from build123d import *

# Parameters (mm, degrees)
SKETCH1_W               = 20.32
SKETCH1_H               = 23.8125
BOSS_EXTRUDE1_DEPTH     = 3
SKETCH3_R               = 1.500000048
CUT_EXTRUDE1_DEPTH      = 84.279291716
CUT_EXTRUDE2_DEPTH      = 23.075453704
CUT_EXTRUDE2_DEPTH_BACK = 23.075453704
SKETCH2_R               = 78.359
SKETCH4_W               = 22.86
SKETCH4_H               = 20.306074834
CUT_EXTRUDE3_DEPTH      = 12.3825
SKETCH9_W               = 8
SKETCH9_H               = 3.175
BOSS_EXTRUDE2_DEPTH     = 10.16
BOSS_EXTRUDE3_DEPTH     = 1.27
FILLET7_R               = 5.715
FILLET8_R               = 1.27
FILLET9_R               = 1.27


# Some blends are built 0.0001 mm under size
with BuildPart() as part:
    # Sketch1 → Boss-Extrude1 (new body)
    with BuildSketch(Plane(origin=(0, 0, 0), x_dir=(1, 0, 0), z_dir=(0, 1, 0))):
        with Locations((0, -7.46125)):
            Rectangle(SKETCH1_W, SKETCH1_H)
        Polygon((3.9, -10.985), (6, -10.985), (6, -13.985), (2.999999969, -13.985), (2.999999969, -17.16), (-2.999999969, -17.16), (-2.999999969, -13.985), (-6, -13.985), (-6, -10.985), (-3.9, -10.985), (-3.9, -6.985), (3.9, -6.985), align=None, mode=Mode.SUBTRACT)
    extrude(amount=BOSS_EXTRUDE1_DEPTH)

    # Sketch3 → Cut-Extrude1 (cut, through all)
    with BuildSketch(Plane(origin=(-5.581860717, -76.451458097, 0), x_dir=(0, 0, 1), z_dir=(0.07281799962939917, 0.9973452456045363, 0))):
        with Locations(Location((0, 5.59671863, 0), (0, 0, 270))):
            Circle(SKETCH3_R)
    cut_extrude1 = extrude(amount=CUT_EXTRUDE1_DEPTH, mode=Mode.SUBTRACT)

    # Mirror1: Cut-Extrude1 across plane
    add(cut_extrude1.mirror(Plane(origin=(0, 0, 0), x_dir=(0, 0, 1), z_dir=(1, 0, 0))), mode=Mode.SUBTRACT)

    # Sketch2 → Cut-Extrude2 (cut, two sides: drawn at the far end of the back side and taken through both)
    with BuildSketch(Plane.XY.offset(-CUT_EXTRUDE2_DEPTH_BACK)):
        with Locations((0, -76.858999952)):
            Circle(SKETCH2_R)
    extrude(amount=CUT_EXTRUDE2_DEPTH + CUT_EXTRUDE2_DEPTH_BACK, mode=Mode.SUBTRACT)

    # Sketch4 → Cut-Extrude3 (cut)
    with BuildSketch(Plane.XY.offset(19.3675)):
        with Locations((-1.27, 10.991574627)):
            Rectangle(SKETCH4_W, SKETCH4_H)
    extrude(amount=-CUT_EXTRUDE3_DEPTH, mode=Mode.SUBTRACT)

    # Sketch9 → Boss-Extrude2 (add)
    with BuildSketch(Plane(origin=(0, 3, 0), x_dir=(1, 0, 0), z_dir=(0, 1, 0))):
        with Locations((0, -5.3975)):
            Rectangle(SKETCH9_W, SKETCH9_H)
    extrude(amount=BOSS_EXTRUDE2_DEPTH)

    # Sketch10 → Boss-Extrude3 (add, symmetric)
    with BuildSketch(Plane(origin=(0, 0, 0), x_dir=(0, 0, -1), z_dir=(1, 0, 0))):
        Polygon((-3.81, 13.16), (4.445, 3), (-3.81, 3), align=None)
    extrude(amount=BOSS_EXTRUDE3_DEPTH, both=True)

    # Fillet7
    fillet7_edges = [part.edges().sort_by_distance(p)[0] for p in [
        (-10.16, 1.919268605, 6.985),
        (-10.16, 1.919268605, -4.445),
        (10.16, 1.919268605, -4.445),
        (10.16, 1.919268605, 6.985),
    ]]
    fillet(fillet7_edges, radius=FILLET7_R - 0.0001)  # a hair under: the kernel refuses the full size

    # Fillet8
    fillet8_edges = [part.edges().sort_by_distance(p)[0] for p in [
        (4, 8.08, 6.985),
        (4, 8.08, 3.81),
        (-4, 8.08, 3.81),
        (-4, 8.08, 6.985),
        (0, 13.16, 6.985),
    ]]
    fillet(fillet8_edges, radius=FILLET8_R)

    # Fillet9
    # the kernel refuses this fillet: 1.27 mm, written as the material it adds along each edge
    with BuildSketch(Plane(origin=(-1.27, 3, 3.81), x_dir=(0, 0, -1), z_dir=(0, 1, 0))) as fillet9_piece_1_section:
        with BuildLine():
            CenterArc((FILLET9_R, FILLET9_R), FILLET9_R, 180, 90)
            Line((0, FILLET9_R), (0, 0))
            Line((0, 0), (FILLET9_R, 0))
        make_face()
    fillet9_piece_1 = extrude(amount=10.16, mode=Mode.PRIVATE)
    fillet9_piece_1 = split(fillet9_piece_1, bisect_by=Plane(origin=(-1.56303802, 9.860421862, 1.129092762), z_dir=(0, -0.630592625094466, 0.7761140001162654)), keep=Keep.TOP, mode=Mode.PRIVATE)
    add(fillet9_piece_1)
    with BuildSketch(Plane(origin=(-1.27, 3, -4.445), x_dir=(-1, 0, 0), z_dir=(0, 0, 1))) as fillet9_piece_2_section:
        with BuildLine():
            CenterArc((FILLET9_R, -FILLET9_R), FILLET9_R, 90, 90)
            Line((0, -FILLET9_R), (0, 0))
            Line((0, 0), (FILLET9_R, 0))
        make_face()
    fillet9_piece_2 = extrude(amount=11.43, mode=Mode.PRIVATE)
    fillet9_piece_2 = split(fillet9_piece_2, bisect_by=Plane(origin=(-1.561973496, 5.244551774, -2.621301684), z_dir=(0, -0.630592625094466, 0.7761140001162654)), keep=Keep.TOP, mode=Mode.PRIVATE)
    add(fillet9_piece_2)
    with BuildSketch(Plane(origin=(1.27, 3, 3.81), x_dir=(0, 0, -1), z_dir=(0, 1, 0))) as fillet9_piece_3_section:
        with BuildLine():
            CenterArc((FILLET9_R, -FILLET9_R), FILLET9_R, 90, 90)
            Line((0, -FILLET9_R), (0, 0))
            Line((0, 0), (FILLET9_R, 0))
        make_face()
    fillet9_piece_3 = extrude(amount=10.16, mode=Mode.PRIVATE)
    fillet9_piece_3 = split(fillet9_piece_3, bisect_by=Plane(origin=(1.56303802, 9.860421862, 1.129092762), z_dir=(0, -0.630592625094466, 0.7761140001162654)), keep=Keep.TOP, mode=Mode.PRIVATE)
    add(fillet9_piece_3)
    with BuildSketch(Plane(origin=(1.27, 3, -4.445), x_dir=(1, 0, 0), z_dir=(0, 0, 1))) as fillet9_piece_4_section:
        with BuildLine():
            CenterArc((FILLET9_R, FILLET9_R), FILLET9_R, 180, 90)
            Line((0, FILLET9_R), (0, 0))
            Line((0, 0), (FILLET9_R, 0))
        make_face()
    fillet9_piece_4 = extrude(amount=11.43, mode=Mode.PRIVATE)
    fillet9_piece_4 = split(fillet9_piece_4, bisect_by=Plane(origin=(1.561973496, 5.244551774, -2.621301684), z_dir=(0, -0.630592625094466, 0.7761140001162654)), keep=Keep.TOP, mode=Mode.PRIVATE)
    add(fillet9_piece_4)


solid = part.part
Geometry check sheet. Reference: the model listing, model coordinates, mm. A direction names the side the tool comes from. Round coordinates to 2 decimals unless told otherwise and drop trailing zeros. Loops run counter-clockwise (first coordinate to the right, second up) from the corner with the lowest first, then second, coordinate; pieces in that order, holes last.
Item 1: Cross-section at C-C on z = 5.5. Record the boundary of the cut face in (x, y).
Item 2: Mould release check, pull along Z, two halves, no side actions. Record for faces 5 (the cylindrical face through (7.266, 2.076, 0.066)), 6 (the cylindrical face through (3.638, 8.151, 4.192)), 7 (the cylindrical face through (1.632, 3.382, -0.375)): pulls with the +Z half, pulls with the -Z half, needs draft (parallel to the pull), parting line crosses it, or undercut.
Item 3: Thickness scan on line 1 (X direction, y = 5.25, z = -2); line 2 (Y direction, x = 6, z = 5); line 3 (Z direction, x = 5, y = 2.25). Record the ranges inside material, lowest first.
Item 4: Cross-section at A-A on z = -0.25. Record the boundary of the cut face in (x, y), then the cut area to 3 significant figures.
Item 5: Cross-section at B-B on y = 9. Record the boundary of the cut face in (x, z) (3 decimals).
Item 6: Gauge pin test, flat ends, axial feed: pin 1 (2.5 mm diameter, centred on x = 7.5, z = 0.5, fed in from +Y); pin 2 (0.5 mm diameter, centred on y = 8, z = 5.5, fed in from -X); pin 3 (1.5 mm diameter, centred on y = 7, z = 3.5, fed in from -X). Record the tip position at first contact, or that the pin passes through.
Item 7: Access from +Z, -Z, +X, -X, +Y, -Y to the whole of each face (thin tool, end or side, straight path). Record for faces 1 (the flat face through (-1.27, 6, 1)), 2 (the cylindrical face through (3.62, 8.15, 6.62)), 3 (the cylindrical face through (-3.62, 8.15, 6.62)), 4 (the cylindrical face through (1.632, 8.009, 3.428)).
Item 8: Cross-section at D-D on x = -2.25. Record the boundary of the cut face in (y, z) (3 decimals).
Answer sheet:
1. outline: (-8.29, 1.06) arc R78.36 cw to (8.29, 1.06) - (8.29, 3) - (4, 3) - (4, 13.16) - (-4, 13.16) - (-4, 3) - (-8.29, 3) - close
2. face 5: undercut
2. face 6: pulls with the -Z half
2. face 7: needs draft
3. line 1: x = -1.27 to 1.27
3. line 2: y = 1.27 to 3
3. line 3: z = -4.42 to -1.28, 1.28 to 6.96
4. outline: (-9.95, 0.87) arc R78.36 cw to (-7.18, 1.17) - (-7.31, 3) - (-9.95, 3) - close; (-4.35, 3) - (-4.23, 1.39) arc R78.36 cw to (4.23, 1.39) - (4.35, 3) - (2.54, 3) arc R1.27 cw to (1.27, 4.27) - (1.27, 8.16) - (-1.27, 8.16) - (-1.27, 4.27) arc R1.27 cw to (-2.54, 3) - close; (7.18, 1.17) arc R78.36 cw to (9.95, 0.87) - (9.95, 3) - (7.31, 3) - close
4. area: 37.7 mm2
5. outline: (-4, 5.08) arc R1.27 ccw to (-2.73, 3.81) - (-2.54, 3.81) arc R1.27 cw to (-1.27, 2.54) - (-1.27, 0.43) - (1.27, 0.43) - (1.27, 2.54) arc R1.27 cw to (2.54, 3.81) - (2.73, 3.81) arc R1.27 ccw to (4, 5.08) - (4, 5.715) arc R1.27 ccw to (2.73, 6.985) - (-2.73, 6.985) arc R1.27 ccw to (-4, 5.715) - close
6. pin 1: stops at y = 3
6. pin 2: stops at x = -4
6. pin 3: stops at x = -3.69
7. face 1: -Z, -X, +Y
7. face 2: +Z, +X, +Y
7. face 3: +Z, -X, +Y
7. face 4: -Z, +X, +Y
8. outline: (1.468, -4.445) - (3, -4.445) - (3.034, -4.418) - (3.034, 3.776) - (13.119, 3.776) - (13.16, 3.81) - (13.16, 5.715) arc R1.27 ccw to (11.89, 6.985) - (1.468, 6.985) - close
